Here's how the part is built. I have some questions about the finished solid (model axes, mm). A direction names the side the tool comes from. Coordinates: 2 decimals unless noted, no trailing zeros. Write each loop counter-clockwise with the first axis right and the second up, starting at its lowest first coordinate (ties: lowest second). Pieces come first, ordered by that corner, then holes.
Item 1: I want a section at A-A (z = 10). Count the separate pieces of the cut face and the enclosed holes in it, and give its area (3 significant figures).
Item 2: If we mould it in two halves opening along Z, with no side actions, what happens to faces 3 (the face through (24, 24, 0)), 4 (the face through (32, 33, 2)), 5 (the face through (2.465, 32.425, 9.189))? For each: pulls with the +Z half, pulls with the -Z half, needs draft (parallel to the pull), parting line crosses it, or undercut.
Item 3: For faces 1 (the face through (30, 0, 10)), 2 (the face through (20, 21, 15)), which set-ups out of +Z, -Z, +X, -X, +Y, -Y let a thin tool reach every point of the face, with its end or its side?
Item 4: I want a section at B-B (x = 15). Please give me the cut outline in (y, z), and give its area (3 significant figures).
Item 5: I want a section at C-C (y = 55). Please give me the cut outline in (x, z), and give its area (3 significant figures).
Item 6: I want a section at D-D (y = 27). Please give me the cut outline in (x, z).
Item 7: I'm going to push flat-ended pins straight in: P1, Ø6, axis at y = 35, z = 10, coming from the +X side; P2, Ø12, axis at y = 31.5, z = 17, coming from the +X side; P3, Ø8, axis at y = 40, z = 12, coming from the +X side. Where does each tip first touch, or does it pass through?
Item 8: Please list where these lines run through material, in increasing order: line 1 (X direction, y = 2.1, z = 10); line 2 (Z direction, x = 15, y = 1.6).
from build123d import *

# Parameters (mm, degrees)
CYLINDER001_R     = 2.7
CYLINDER001_DEPTH = 5
CYLINDER002_R     = 2.7
CYLINDER002_DEPTH = 5
CYLINDER004_R     = 2.7
CYLINDER004_DEPTH = 5
CYLINDER003_R     = 2.7
CYLINDER003_DEPTH = 5
CYLINDER005_R     = 2.7
CYLINDER005_DEPTH = 5
CYLINDER_R        = 2.7
CYLINDER_DEPTH    = 5
PAD_DEPTH         = 5
PAD001_DEPTH      = 10
PAD002_DEPTH      = 5


with BuildPart() as cylinder001:
    # Cylinder001 → Cylinder001 (new body)
    with BuildSketch(Plane(origin=(55, 0, 10), x_dir=(1, 0, 0), z_dir=(0, 1, 0))):
        Circle(CYLINDER001_R)
    extrude(amount=CYLINDER001_DEPTH)


with BuildPart() as cylinder002:
    # Cylinder002 → Cylinder002 (new body)
    with BuildSketch(Plane(origin=(0, 15, 10), x_dir=(0, -1, 0), z_dir=(1, 0, 0))):
        Circle(CYLINDER002_R)
    extrude(amount=CYLINDER002_DEPTH)


with BuildPart() as cylinder004:
    # Cylinder004 → Cylinder004 (new body)
    with BuildSketch(Plane(origin=(35, 0, 10), x_dir=(1, 0, 0), z_dir=(0, 1, 0))):
        Circle(CYLINDER004_R)
    extrude(amount=CYLINDER004_DEPTH)


with BuildPart() as cylinder003:
    # Cylinder003 → Cylinder003 (new body)
    with BuildSketch(Plane(origin=(0, 55, 10), x_dir=(0, -1, 0), z_dir=(1, 0, 0))):
        Circle(CYLINDER003_R)
    extrude(amount=CYLINDER003_DEPTH)


with BuildPart() as cylinder005:
    # Cylinder005 → Cylinder005 (new body)
    with BuildSketch(Plane(origin=(0, 35, 10), x_dir=(0, -1, 0), z_dir=(1, 0, 0))):
        Circle(CYLINDER005_R)
    extrude(amount=CYLINDER005_DEPTH)


with BuildPart() as compound:
    # Cylinder → Cylinder (new body)
    with BuildSketch(Plane(origin=(15, 0, 10), x_dir=(1, 0, 0), z_dir=(0, 1, 0))):
        Circle(CYLINDER_R)
    extrude(amount=CYLINDER_DEPTH)

    # Compound: union Cylinder001, Cylinder002, Cylinder004, Cylinder003, Cylinder005
    add(cylinder001.part)
    add(cylinder002.part)
    add(cylinder004.part)
    add(cylinder003.part)
    add(cylinder005.part)


with BuildPart() as f_60mm_bracket:
    # Sketch → Pad (new body)
    with BuildSketch(Plane.XY):
        Polygon((0, 0), (0, 60), (5, 60), (60, 5), (60, 0), align=None)
    extrude(amount=PAD_DEPTH)

    # Sketch001 (on Face7 of Pad) → Pad001 (join)
    with BuildSketch(Plane.XY.offset(5)):
        Polygon((0, 60), (0, 0), (60, 0), (60, 5), (5, 5), (5, 60), align=None)
    extrude(amount=PAD001_DEPTH)

    # Sketch002 (on Face10 of Pad001) → Pad002 (join)
    with BuildSketch(Plane.XY.offset(15)):
        Polygon((0, 60), (0, 0), (60, 0), (60, 5), (5, 60), align=None)
    extrude(amount=PAD002_DEPTH)

    # Cut: cut Compound
    add(compound.part, mode=Mode.SUBTRACT)


solid = f_60mm_bracket.part
Answer:
1. separate pieces: 7
1. enclosed holes: 0
1. area: 413 mm2
2. face 3: pulls with the -Z half
2. face 4: needs draft
2. face 5: undercut
3. face 1: +Z, -Z, +X, -X, -Y
3. face 2: +X, +Y
4. outline: (0, 0) - (50, 0) - (50, 5) - (5, 5) - (5, 7.3) - (0, 7.3) - close; (0, 12.7) - (5, 12.7) - (5, 15) - (50, 15) - (50, 20) - (0, 20) - close
4. area: 523 mm2
5. outline: (0, 0) - (10, 0) - (10, 5) - (5, 5) - (5, 7.3) - (0, 7.3) - close; (0, 12.7) - (5, 12.7) - (5, 15) - (10, 15) - (10, 20) - (0, 20) - close
5. area: 123 mm2
6. outline: (0, 0) - (38, 0) - (38, 5) - (5, 5) - (5, 15) - (38, 15) - (38, 20) - (0, 20) - close
7. P1: stops at x = 5
7. P2: stops at x = 39.5
7. P3: stops at x = 27.65
8. line 1: x = 0 to 12.3, 17.7 to 32.3, 37.7 to 52.3, 57.7 to 60
8. line 2: z = 0 to 7.3, 12.7 to 20
